The figure shows three views and two pictorial views of one solid part (mm, origin at its lowest corner). Answer the questions. A direction names the side the tool comes from. Give positions to 0.01 mm unless a question says otherwise; leave off trailing zeros. Order: outer loops, then holes, each group sorted by start corner. A loop starts at its lowest first (then second) coordinate and runs counter-clockwise, first axis right, second up. Notation, with made-up numbers: M 56,85.25 L 65,85.25 A16 ccw 65,108.25 Z; hole C 53,72 d5. An arc over 180 degrees is marked long. One line per item, written item: value.
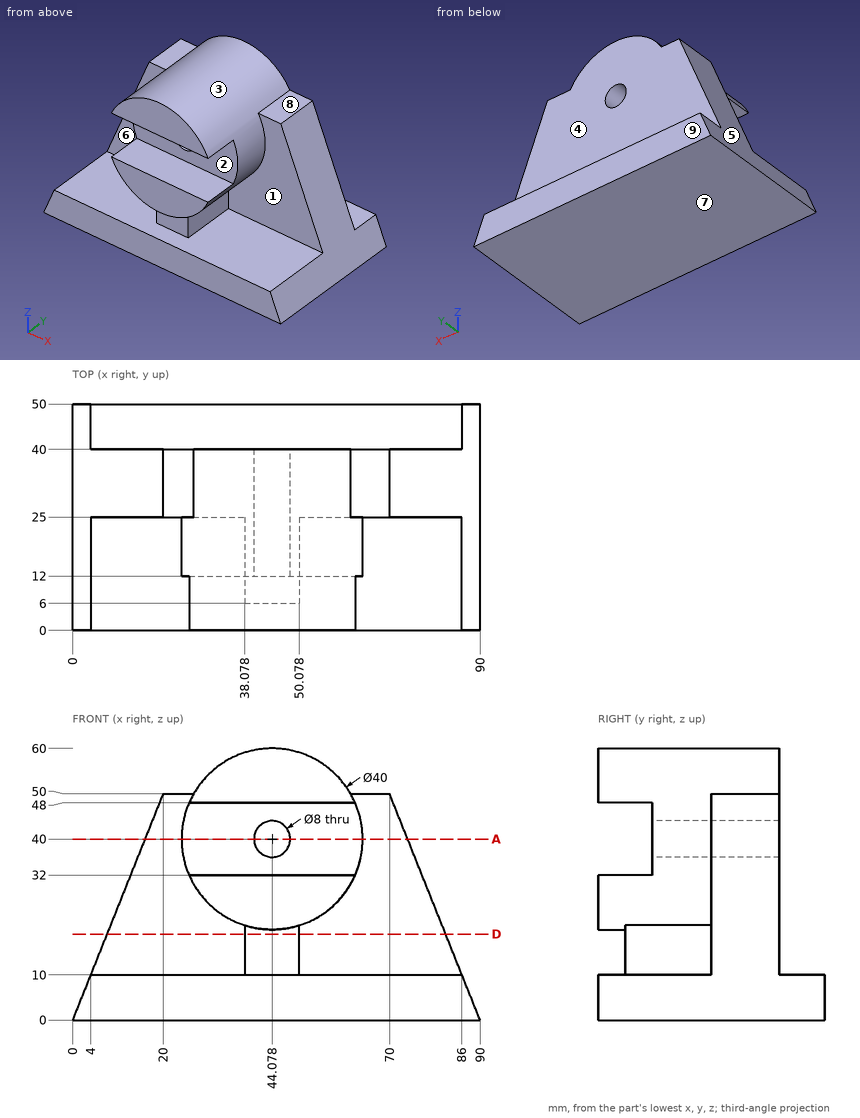
1) Each of these flat-tipped pins is pushed along its axis until it touches: pin 1 Ø12 at (y, z) = (20, 17) entering from +X; pin 2 Ø1.5 at (x, y) = (61, 11) entering from +Z; pin 3 Ø2 at (y, z) = (12.5, 22.5) entering from +X. Where does it stop, or does it pass through?
Reported:
pin 1: stops at x = 84.53
pin 2: stops at z = 51.77
pin 3: stops at x = 55.38
2) Determine the mould class of the marked faces 6, 7, 8 and 9 for opening direction Z: +Z half, -Z half, draft (parallel to the pull), parting line (faces both ways), or undercut.
Reported:
face 6: undercut
face 7: -Z half
face 8: +Z half
face 9: draft
3) Find section A-A, the plane z = 40. Write down the section's boundary in (x, y), plus the area to 3 significant figures.
Reported:
outline: M 16,25 L 24.08,25 L 24.08,12 L 40.08,12 L 40.08,40 L 16,40 Z; M 48.08,12 L 64.08,12 L 64.08,25 L 74,25 L 74,40 L 48.08,40 Z
area: 1,170 mm^2
4) Find section D-D, the plane z = 19. Write down the section's boundary in (x, y), plus the area to 3 significant figures.
Reported:
outline: M 7.6,25 L 38.08,25 L 38.08,6 L 50.08,6 L 50.08,25 L 82.4,25 L 82.4,40 L 7.6,40 Z
area: 1,350 mm^2
5) Consider probe 1 along Y at (x, z) = (10, 19); probe 2 along X at (y, z) = (12.5, 19); probe 3 along Z at (x, y) = (85.5, 18). Determine where each line is inside the solid, lowest interval first.
Reported:
probe 1: y = 25 to 40
probe 2: x = 38.08 to 50.08
probe 3: z = 0 to 10
6) Which of the six approach directions +Z, -Z, +X, -X, +Y, -Y give full straight-line access (tool end or side, diameter ignored) to the marked faces 1, 2, 3, 4 and 5?
Reported:
face 1: +X, -Y
face 2: +X, -X, -Y
face 3: -Y
face 4: +Z, +X, -X, +Y
face 5: +Z, -X, +Y, -Y
